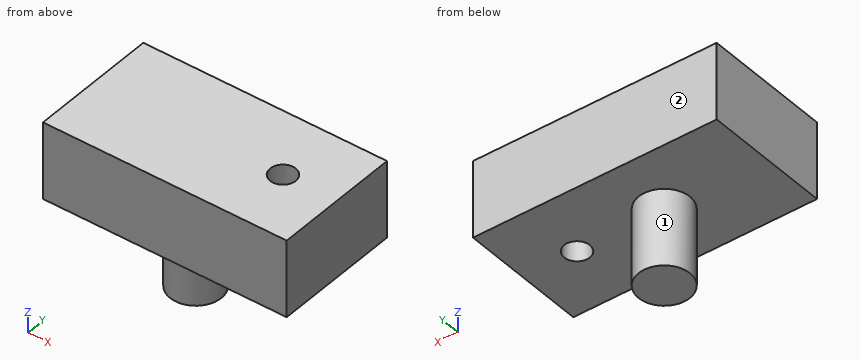
```python
from build123d import *

# Parameters (mm, degrees)
F0_W     = 47.5
F0_H     = 25
F0_R     = 5
F0_R_2   = 2.5
F1_DEPTH = 15
F2_DEPTH = 15


with BuildPart() as f1:
    # F0 (on Top) → F1 (new body)
    with BuildSketch(Plane.XY):
        with Locations((49.75, 50)):
            Rectangle(F0_W, F0_H)
        with Locations((46, 50)):
            Circle(F0_R, mode=Mode.SUBTRACT)
        with Locations((63, 50)):
            Circle(F0_R_2, mode=Mode.SUBTRACT)
        with Locations((46, 50)):
            Circle(F0_R)
    extrude(amount=F1_DEPTH)

    # F0 (on Top) → F2 (join)
    with BuildSketch(Plane.XY):
        with Locations((46, 50)):
            Circle(F0_R)
    extrude(amount=-F2_DEPTH)


solid = f1.part
```
Read the model definition and answer for the solid it produces. Units are mm, in the model's axes. Face numbers are marked on the shaded views. A direction names the side the tool comes from. Give positions to 0.01 mm unless a question says otherwise; leave off trailing zeros. Write each loop counter-clockwise with the first axis right and the second up, starting at its lowest first coordinate (ties: lowest second). Pieces come first, ordered by that corner, then holes. Notation, with made-up numbers: (45.5, 84.25) - (52.5, 84.25) arc R13 ccw to (52.5, 93.25) - close; hole circle Ø7 at (81, 72). An arc over 180 degrees is marked (long way). Write item = value, one per line. Start each with the question number.
Item 1: Find section D-D (y = 46). Give the vertices of the cut face in (x, z).
Item 2: Find section C-C (z = 5.5). Give the vertices of the cut face in (x, y).
Item 3: Find the intervals of material crossed by probe 1 along Y at (x, z) = (63, 4.75); probe 2 along Z at (x, y) = (42, 44.5); probe 3 along X at (y, z) = (51.25, 8), in increasing order. Write a range as [from, to].
Item 4: Find section B-B (y = 50). Give the vertices of the cut face in (x, z).
Item 5: A tool of negligible diameter and unlimited length cuts with its end or side. For the marked faces 1 and 2, from which of +Z, -Z, +X, -X, +Y, -Y can it reach the whole face along a straight path? Write none if from no direction.
Item 6: Find section A-A (x = 63). Give the vertices of the cut face in (y, z), then the cut area to 3 significant figures.
Item 7: Each of these flat-tipped pins is pushed along its axis until it touches: P1, Ø8, axis at x = 63, y = 50, coming from the -Z side; P2, Ø1, axis at y = 47, z = -7, coming from the -X side. Where does it stop, or does it pass through?
Response:
q1.outline = (26, 0) - (43, 0) - (43, -15) - (49, -15) - (49, 0) - (73.5, 0) - (73.5, 15) - (26, 15) - close
q2.outline = (26, 37.5) - (73.5, 37.5) - (73.5, 62.5) - (26, 62.5) - close; hole circle Ø5 at (63, 50)
q3.probe_1 = [37.5, 47.5], [52.5, 62.5]
q3.probe_2 = [0, 15]
q3.probe_3 = [26, 60.83], [65.17, 73.5]
q4.outline = (26, 0) - (41, 0) - (41, -15) - (51, -15) - (51, 0) - (60.5, 0) - (60.5, 15) - (26, 15) - close; (65.5, 0) - (73.5, 0) - (73.5, 15) - (65.5, 15) - close
q5.face_1 = -Z
q5.face_2 = +Z, -Z, +X, -X, +Y
q6.outline = (37.5, 0) - (47.5, 0) - (47.5, 15) - (37.5, 15) - close; (52.5, 0) - (62.5, 0) - (62.5, 15) - (52.5, 15) - close
q6.area = 300 mm²
q7.P1 = 0
q7.P2 = 41.67
